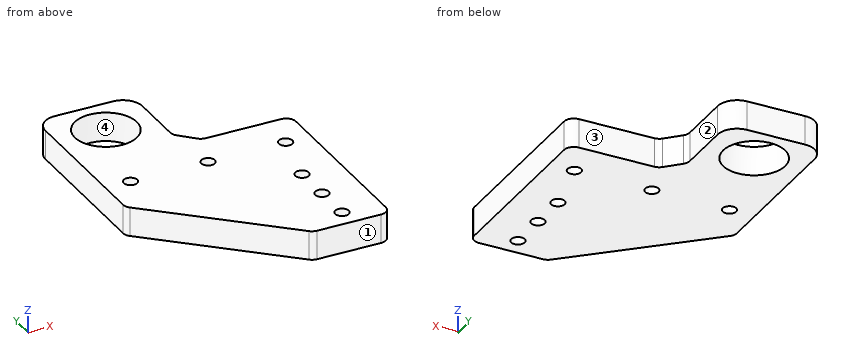
from build123d import *

# Parameters (mm, degrees)
BOSS_EXTRU_1_DEPTH           = 15
ENL_V_MAT_EXTRU_1_DEPTH      = 147.495733726
ENL_V_MAT_EXTRU_1_DEPTH_BACK = 147.495733726
ESQUISSE2_R                  = 3.5
ESQUISSE3_W                  = 50
ESQUISSE3_H                  = 50
BOSS_EXTRU_2_DEPTH           = 15
CHANFREIN1_SIZE              = 10
ENL_V_MAT_EXTRU_2_DEPTH      = 185.285105204
ENL_V_MAT_EXTRU_2_DEPTH_BACK = 185.285105204
ESQUISSE4_R                  = 16
CONG_2_R                     = 5
CONG_3_R                     = 10


with BuildPart() as part:
    # Esquisse1 → Boss.-Extru.1 (new body)
    with BuildSketch(Plane.XY):
        Polygon((0, 0), (0, 100), (-106, 100), (-106, 60), (-40, 0), align=None)
    extrude(amount=BOSS_EXTRU_1_DEPTH)

    # Esquisse2 → Enlèv. mat.-Extru.1 (cut, two sides: drawn at the far end of the back side and taken through both)
    with BuildSketch(Plane.XY.offset(15).offset(-ENL_V_MAT_EXTRU_1_DEPTH_BACK)):
        with Locations((-20, 10)):
            Circle(ESQUISSE2_R)
        with Locations((-20, 30)):
            Circle(ESQUISSE2_R)
        with Locations((-20, 50)):
            Circle(ESQUISSE2_R)
        with Locations((-53, 80)):
            Circle(ESQUISSE2_R)
        with Locations((-93, 80)):
            Circle(ESQUISSE2_R)
        with Locations((-13, 80)):
            Circle(ESQUISSE2_R)
    extrude(amount=ENL_V_MAT_EXTRU_1_DEPTH + ENL_V_MAT_EXTRU_1_DEPTH_BACK, mode=Mode.SUBTRACT)

    # Esquisse3 → Boss.-Extru.2 (add)
    with BuildSketch(Plane.XY.offset(15)):
        with Locations((-81, 125)):
            Rectangle(ESQUISSE3_W, ESQUISSE3_H)
    extrude(amount=-BOSS_EXTRU_2_DEPTH)

    # Chanfrein1
    chanfrein1_edges = [part.edges().sort_by_distance(p)[0] for p in [
        (-56, 100, 7.5),
    ]]
    chamfer(chanfrein1_edges, length=CHANFREIN1_SIZE)

    # Esquisse4 → Enlèv. mat.-Extru.2 (cut, two sides: drawn at the far end of the back side and taken through both)
    with BuildSketch(Plane.XY.offset(15).offset(-ENL_V_MAT_EXTRU_2_DEPTH_BACK)):
        with Locations((-81, 128)):
            Circle(ESQUISSE4_R)
    extrude(amount=ENL_V_MAT_EXTRU_2_DEPTH + ENL_V_MAT_EXTRU_2_DEPTH_BACK, mode=Mode.SUBTRACT)

    # Congé2
    cong_2_edges = [part.edges().sort_by_distance(p)[0] for p in [
        (-46, 100, 7.5),
        (-56, 110, 7.5),
        (-40, 0, 7.5),
        (-106, 60, 7.5),
        (0, 100, 7.5),
        (0, 0, 7.5),
    ]]
    fillet(cong_2_edges, radius=CONG_2_R)

    # Congé3
    cong_3_edges = [part.edges().sort_by_distance(p)[0] for p in [
        (-106, 150, 7.5),
        (-56, 150, 7.5),
    ]]
    fillet(cong_3_edges, radius=CONG_3_R)


solid = part.part
The listing builds one solid part. Answer for the finished solid, in the listing's coordinates (mm). Face numbers are marked on the shaded views. Coordinates: 2 decimals unless noted, no trailing zeros. Write each loop counter-clockwise with the first axis right and the second up, starting at its lowest first coordinate (ties: lowest second). Pieces come first, ordered by that corner, then holes. Notation, with made-up numbers: (17.5, -5) -> (56.5, -5) arc R33 cw to (56.5, 28) -> close; hole circle Ø4 at (8.5, 41.5). An arc over 180 degrees is marked (long way). One line per question, with ' | ' between items.
1. Section C-C (y = 80) is taken. Determine the outline of the cut face in (x, z).
Verdict:
outline: (-106, 0) -> (-96.5, 0) -> (-96.5, 15) -> (-106, 15) -> close; (-89.5, 0) -> (-56.5, 0) -> (-56.5, 15) -> (-89.5, 15) -> close; (-49.5, 0) -> (-16.5, 0) -> (-16.5, 15) -> (-49.5, 15) -> close; (-9.5, 0) -> (0, 0) -> (0, 15) -> (-9.5, 15) -> close
2. Straight lines are drawn through the part: line 1 (Y direction, x = -20, z = 9.25); line 2 (X direction, y = 128, z = 4.75); line 3 (X direction, y = 77, z = 7.5). For each, find the intervals that lie inside material, in ascending order.
Verdict:
line 1: y = 0 to 6.5, 13.5 to 26.5, 33.5 to 46.5, 53.5 to 100 | line 2: x = -106 to -97, -65 to -56 | line 3: x = -106 to -94.8, -91.2 to -54.8, -51.2 to -14.8, -11.2 to 0
3. Section A-A (y = 50) is taken. Determine the outline of the cut face in (x, z), and give its area (3 significant figures).
Verdict:
outline: (-95, 0) -> (-23.5, 0) -> (-23.5, 15) -> (-95, 15) -> close; (-16.5, 0) -> (0, 0) -> (0, 15) -> (-16.5, 15) -> close | area: 1,320 mm^2
4. Section B-B (x = -20) is taken. Determine the outline of the cut face in (y, z).
Verdict:
outline: (0, 0) -> (6.5, 0) -> (6.5, 15) -> (0, 15) -> close; (13.5, 0) -> (26.5, 0) -> (26.5, 15) -> (13.5, 15) -> close; (33.5, 0) -> (46.5, 0) -> (46.5, 15) -> (33.5, 15) -> close; (53.5, 0) -> (100, 0) -> (100, 15) -> (53.5, 15) -> close
5. Given pin 1 Ø4 at (x, y) = (-20, 50) entering from +Z; pin 2 Ø2 at (x, z) = (-31.5, 13) entering from +Y; pin 3 Ø6 at (x, z) = (-67, 12.5) entering from -Y, each flat-ended and moving along its own axis, determine where each tip first touches the part or whether it passes through.
Verdict:
pin 1: passes through | pin 2: stops at y = 100 | pin 3: stops at y = 21.82
6. For a pull along Y with two mould halves and no side action, classify the marked faces 1, 2, 3 and 4 as released by +Y, released by -Y, zero draft, split by the parting line, or undercut.
Verdict:
face 1: released by -Y | face 2: zero draft | face 3: released by +Y | face 4: undercut
7. Section D-D (z = 9.5) is taken. Determine the outline of the cut face in (x, y).
Verdict:
outline: (-106, 62.21) arc R5 ccw to (-104.36, 58.51) -> (-41.43, 1.3) arc R5 ccw to (-38.07, 0) -> (-5, 0) arc R5 ccw to (0, 5) -> (0, 95) arc R5 ccw to (-5, 100) -> (-43.93, 100) arc R5 cw to (-47.46, 101.46) -> (-54.54, 108.54) arc R5 cw to (-56, 112.07) -> (-56, 140) arc R10 ccw to (-66, 150) -> (-96, 150) arc R10 ccw to (-106, 140) -> close; hole circle Ø32 at (-81, 128); hole circle Ø7 at (-93, 80); hole circle Ø7 at (-53, 80); hole circle Ø7 at (-20, 10); hole circle Ø7 at (-20, 30); hole circle Ø7 at (-20, 50); hole circle Ø7 at (-13, 80)
